Autodesk Inventor part; units mm, degrees
sketch "スケッチ1" plane through (0, 0, 0) normal (0, 0, 1) x (1, 0, 0)
  line L0 (-21.5, 10.75) -> (21.5, 10.75)
  line L1 (21.5, 10.75) -> (21.5, -10.75)
  line L2 (21.5, -10.75) -> (-21.5, -10.75)
  line L3 (-21.5, -10.75) -> (-21.5, 10.75)
  line L4 (-21.5, -10.75) -> (21.5, 10.75)
  line L5 (-21.5, 10.75) -> (21.5, -10.75)
  point P0 (0, 0)
  dimension "d0" = 43
  dimension "d1" = 21.5
extrude "押し出し1" add sketch "スケッチ1" along normal blind 1.4
sketch "スケッチ2" plane through (0, 0, 0) normal (0, 0, -1) x (-1, 0, 0)
  circle A0 centre (-15, -8.25) radius 1.5
  point P0 (0, 0)
  dimension "d4" = 3
  dimension "d5" = 15
  dimension "d6" = 8.25
extrude "押し出し2" cut sketch "スケッチ2" against normal through all
sketch "スケッチ3" plane through (0, 0, 0) normal (0, 0, -1) x (-1, 0, 0)
  circle A0 centre (-17, 0) radius 4
  line L0 (-2, -9) -> (-12, -9)
  line L1 (-12, -9) -> (-12, 1)
  line L2 (-12, 1) -> (-2, 1)
  line L3 (-2, 1) -> (-2, -9)
  point P0 (0, 0)
  dimension "d12" = 8
  dimension "d13" = 17
  dimension "d16" = 10
  dimension "d17" = 10
  dimension "d18" = 2
  dimension "d23" = 1
extrude "押し出し3" add sketch "スケッチ3" against normal blind 11.8
pattern_circular "円形状パターン2" count 2 over 360 about axis through (0, 0, -10) along (0, 0, 1) of "押し出し3", "押し出し2"
sketch "スケッチ4" plane through (0, 0, 0) normal (0, 0, -1) x (-1, 0, 0)
  line L0 (-2.2, 4.45) -> (-11.7, 4.45)
  line L1 (-11.7, 4.45) -> (-11.7, 9.25)
  line L2 (-11.7, 9.25) -> (-2.2, 9.25)
  line L3 (-2.2, 9.25) -> (-2.2, 4.45)
  circle A0 centre (15, 8.25) radius 1.5
  circle A1 centre (-15, -8.25) radius 1.5
  line L4 (21.5, -10.75) -> (-21.5, -10.75)
  line L5 (21.5, 10.75) -> (21.5, -10.75)
  line L6 (-21.5, 10.75) -> (21.5, 10.75)
  line L7 (-21.5, -10.75) -> (-21.5, 10.75)
  point P0 (0, 0)
  dimension "d24" = 9.5
  dimension "d25" = 4.8
  dimension "d26" = 1.5
  dimension "d27" = 9.8
extrude "押し出し4" add sketch "スケッチ4" against normal blind 11.3 contours L0 L1 L2 L3
sketch "スケッチ5" plane through (0, 0, 11.3) normal (0, 0, 1) x (1, 0, 0)
  line L0 (2.2, 4.45) -> (11.7, 4.45)
  line L1 (11.7, 4.45) -> (11.7, 9.25)
  line L2 (11.7, 9.25) -> (2.2, 9.25)
  line L3 (2.2, 9.25) -> (2.2, 4.45)
  circle A0 centre (3.3, 8.15) radius 1.1
  point P0 (0, 0)
  dimension "d30" = 2.2
extrude "押し出し5" add sketch "スケッチ5" along normal blind 1.5 contours A0
move faces "移動1" translate (0, 0, -3) faces at (8.6667, -2.3333, 11.8)
move faces "移動2" translate (0, 0, -5.9) faces at (-5.3333, 5.6667, 11.8)
properties part number "DC-DCconverter"
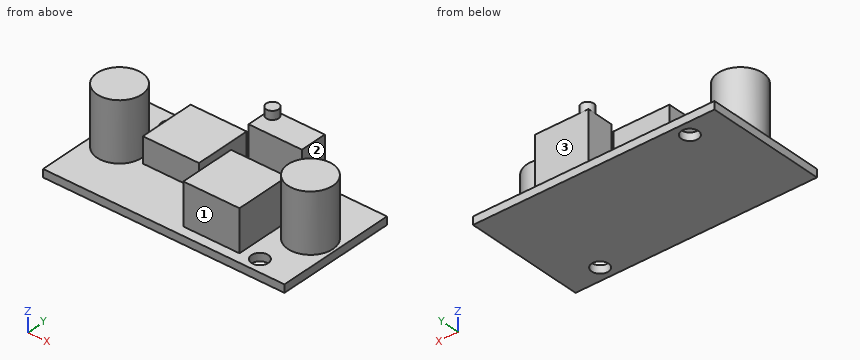
Geometry check sheet. Reference: the model listing, model coordinates, mm. Face numbers are marked on the shaded views. A direction names the side the tool comes from. Coordinates: 2 decimals unless noted, no trailing zeros. Write each loop counter-clockwise with the first axis right and the second up, starting at its lowest first coordinate (ties: lowest second). Pieces come first, ordered by that corner, then holes. Notation, with made-up numbers: M -32,-5 L -13,-5 A32 cw -13,22 Z; hole C 78,32 d11. An arc over 180 degrees is marked long. Answer as a JSON object with one key per item and string values.
1. Tool access check on the marked faces 1, 2 and 3. Record the directions out of +Z, -Z, +X, -X, +Y, -Y that give a thin tool (end or side, any length) a straight path to the whole face; none if there is none.
Answers below:
{"face 1": "+Z, +X, -X, -Y", "face 2": "+Z, +X, +Y", "face 3": "+Z, +X, -X, +Y"}
2. Section check C-C, the plane x = 17. Enter the section's corners in (y, z).
Answers below:
{"outline": "M -10.75,0 L 10.75,0 L 10.75,1.4 L 4,1.4 L 4,11.8 L -4,11.8 L -4,1.4 L -10.75,1.4 Z"}
3. Go/stop test with flat-tipped pins: pin 1 Ø2.5 at (x, y) = (-18, 0) entering from +Z; pin 2 Ø1.8 at (x, y) = (15, -8.25) entering from -Z; pin 3 Ø2 at (x, z) = (7.5, 6) entering from -Y; pin 4 Ø3 at (y, z) = (-7, 7) entering from -X. Record where each tip stops, or that it passes through.
Answers below:
{"pin 1": "stops at z = 11.8", "pin 2": "passes through", "pin 3": "stops at y = -9", "pin 4": "stops at x = 2"}
4. Scan lines: L1, parallel to Y at x = 15, z = 0.6; L2, parallel to Y at x = -15, z = 0.6; L3, parallel to X at y = 8.25, z = 1. Record each from-to range of solid material in increasing order.
Answers below:
{"L1": "y = -10.75 to -9.75, -6.75 to 10.75", "L2": "y = -10.75 to 6.75, 9.75 to 10.75", "L3": "x = -21.5 to -16.5, -13.5 to 21.5"}
5. Section check A-A, the plane z = 8.25. Enter the section's corners in (x, y).
Answers below:
{"outline": "C -17,0 d8; M 2,-9 L 12,-9 L 12,1 L 2,1 Z; M 2.2,4.45 L 11.7,4.45 L 11.7,9.25 L 2.2,9.25 Z; C 17,0 d8"}
6. Section check D-D, the plane z = 1. Enter the section's corners in (x, y).
Answers below:
{"outline": "M -21.5,-10.75 L 21.5,-10.75 L 21.5,10.75 L -21.5,10.75 Z; hole C -15,8.25 d3; hole C 15,-8.25 d3"}
7. Section check B-B, the plane y = -8.25. Enter the section's corners in (x, z), plus the area to 3 significant figures.
Answers below:
{"outline": "M -21.5,0 L 13.5,0 L 13.5,1.4 L 12,1.4 L 12,8.8 L 2,8.8 L 2,1.4 L -21.5,1.4 Z; M 16.5,0 L 21.5,0 L 21.5,1.4 L 16.5,1.4 Z", "area": "130 mm²"}
